Design review of the part built by this model. Coordinates are the model's own, in mm. Face numbers are marked on the shaded views. A direction names the side the tool comes from. Coordinates: 2 decimals unless noted, no trailing zeros. Write each loop counter-clockwise with the first axis right and the second up, starting at its lowest first coordinate (ties: lowest second). Pieces come first, ordered by that corner, then holes. Notation, with made-up numbers: (75.25, 30.25) -> (118.25, 30.25) arc R22 cw to (118.25, 42.25) -> close; hole circle Ø3 at (26.5, 11.25). An arc over 180 degrees is marked (long way). Answer in a Markdown table with one row per item. Add a question column.
Item 1: Clearance check with flat-ended pins moving along their axes: P1, Ø5.5, axis at x = -1.5, y = -1.5, coming from the +Z side; P2, Ø11, axis at x = -1.5, y = -0.5, coming from the +Z side. State where each tip first meets the part, or that it passes through.
Item 2: Take a section at A-A, the plane y = 1.75. Write out the cut boundary in (x, z).
Item 3: For the marked faces 4 and 5, list the 3-axis set-ups (+Z, -Z, +X, -X, +Y, -Y) from which the entire face can be reached by the end or side of a thin tool; tool diameter is ignored.
Item 4: Take a section at C-C, the plane z = 10.55. Write out the cut boundary in (x, y), and give its area (3 significant figures).
Item 5: Take a section at B-B, the plane x = 20. Write out the cut boundary in (y, z).
Item 6: Take a section at D-D, the plane z = 4. Write out the cut boundary in (x, y).
Item 7: To check wall thickness, follow line 1 (X direction, y = 0, z = -15); line 2 (X direction, y = -10.5, z = -3); line 3 (Y direction, x = 0.5, z = -14). State the ranges of each line that lie inside material, in increasing order.
Item 8: Draft analysis for pull direction Y (two halves, no side actions). For the marked faces 1, 2 and 3, state which applies: released by +Y, released by -Y, zero draft, split by the parting line, or undercut.
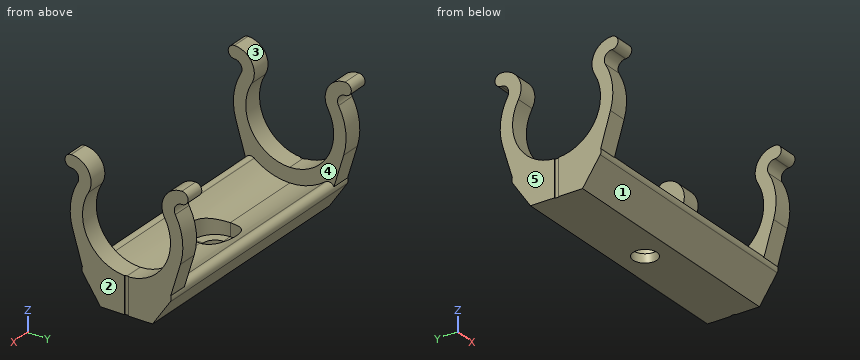
from build123d import *

# Parameters (mm, degrees)
PAD005_DEPTH                  = 29
PAD006_DEPTH                  = 4.5
SKETCH014_R                   = 2.75
POCKET005_DEPTH               = 107.300407
SKETCH015_R                   = 5
POCKET006_DEPTH               = 16.5
PAD005_MIRRORED002_2_DEPTH    = 29
PAD006_MIRRORED002_2_DEPTH    = 4.5
SKETCH014_MIRRORED002_2_R     = 2.75
POCKET005_MIRRORED002_2_DEPTH = 107.300407
SKETCH015_MIRRORED002_2_R     = 5
POCKET006_MIRRORED002_2_DEPTH = 16.5
SKETCH023_W                   = 1
SKETCH023_H                   = 10
POCKET011_DEPTH               = 0.2


with BuildPart() as part:
    # Sketch012 → Pad005 (new body)
    with BuildSketch(Plane.YZ):
        with BuildLine():
            ThreePointArc((0, -13.5), (4.330629, -12.786542), (8.203522, -10.721578))
            ThreePointArc((10.083563, -12.5), (9.900722, -10.810344), (8.203522, -10.721578))
            Line((6, -18.5), (10.083563, -12.5))
            Line((0, -18.5), (6, -18.5))
            Line((0, -13.5), (0, -18.5))
        make_face()
    pad005 = extrude(amount=PAD005_DEPTH)

    # Sketch013 → Pad006 (join)
    with BuildSketch(Plane.YZ.offset(29)):
        with BuildLine():
            ThreePointArc((0, -10.15), (8.790158, -5.075), (8.790158, 5.075))
            ThreePointArc((12.773875, 11.975), (8.790158, 9.675), (8.790158, 5.075))
            ThreePointArc((12.773875, 9.125), (14.198875, 10.55), (12.773875, 11.975))
            ThreePointArc((12.773875, 9.125), (11.25833, 8.25), (11.25833, 6.5))
            ThreePointArc((12.442941, -3.764734), (12.914285, 1.490384), (11.25833, 6.5))
            Line((12.442941, -3.764734), (9.8, -12.5))
            Line((9.8, -12.5), (0, -14.15))
            Line((0, -10.15), (0, -14.15))
        make_face()
    pad006 = extrude(amount=-PAD006_DEPTH)

    # Sketch014 → Pocket005 (cut, through all)
    with BuildSketch(Plane.XY):
        Circle(SKETCH014_R)
    pocket005 = extrude(amount=-POCKET005_DEPTH, mode=Mode.SUBTRACT)

    # Sketch015 → Pocket006 (cut)
    with BuildSketch(Plane.XY):
        Circle(SKETCH015_R)
    pocket006 = extrude(amount=-POCKET006_DEPTH, mode=Mode.SUBTRACT)

    # Sketch012 Mirrored002 2 → Pad005 Mirrored002 2 (add)
    with BuildSketch(Plane(origin=(0, 0, 0), x_dir=(0, -1, 0), z_dir=(-1, 0, 0))):
        with BuildLine():
            ThreePointArc((0, -13.5), (4.330629, -12.786542), (8.203522, -10.721578))
            ThreePointArc((10.083563, -12.5), (9.900722, -10.810344), (8.203522, -10.721578))
            Line((6, -18.5), (10.083563, -12.5))
            Line((0, -18.5), (6, -18.5))
            Line((0, -13.5), (0, -18.5))
        make_face()
    pad005_mirrored002_2 = extrude(amount=-PAD005_MIRRORED002_2_DEPTH)

    # Sketch013 Mirrored002 2 → Pad006 Mirrored002 2 (add)
    with BuildSketch(Plane(origin=(29, 0, 0), x_dir=(0, -1, 0), z_dir=(-1, 0, 0))):
        with BuildLine():
            ThreePointArc((0, -10.15), (8.790158, -5.075), (8.790158, 5.075))
            ThreePointArc((12.773875, 11.975), (8.790158, 9.675), (8.790158, 5.075))
            ThreePointArc((12.773875, 9.125), (14.198875, 10.55), (12.773875, 11.975))
            ThreePointArc((12.773875, 9.125), (11.25833, 8.25), (11.25833, 6.5))
            ThreePointArc((12.442941, -3.764734), (12.914285, 1.490384), (11.25833, 6.5))
            Line((12.442941, -3.764734), (9.8, -12.5))
            Line((9.8, -12.5), (0, -14.15))
            Line((0, -10.15), (0, -14.15))
        make_face()
    pad006_mirrored002_2 = extrude(amount=PAD006_MIRRORED002_2_DEPTH)

    # Sketch014 Mirrored002 2 → Pocket005 Mirrored002 2 (cut, through all)
    with BuildSketch(Plane(origin=(0, 0, 0), x_dir=(1, 0, 0), z_dir=(0, 0, -1))):
        Circle(SKETCH014_MIRRORED002_2_R)
    pocket005_mirrored002_2 = extrude(amount=POCKET005_MIRRORED002_2_DEPTH, mode=Mode.SUBTRACT)

    # Sketch015 Mirrored002 2 → Pocket006 Mirrored002 2 (cut)
    with BuildSketch(Plane(origin=(0, 0, 0), x_dir=(1, 0, 0), z_dir=(0, 0, -1))):
        Circle(SKETCH015_MIRRORED002_2_R)
    pocket006_mirrored002_2 = extrude(amount=POCKET006_MIRRORED002_2_DEPTH, mode=Mode.SUBTRACT)

    # Mirrored003: Pad005, Pad006, Pocket005, Pocket006, Pad005 Mirrored002 2, Pad006 Mirrored002 2, Pocket005 Mirrored002 2, Pocket006 Mirrored002 2 across YZ
    add(pad005.mirror(Plane.YZ))
    add(pad006.mirror(Plane.YZ))
    add(pocket005.mirror(Plane.YZ), mode=Mode.SUBTRACT)
    add(pocket006.mirror(Plane.YZ), mode=Mode.SUBTRACT)
    add(pad005_mirrored002_2.mirror(Plane.YZ))
    add(pad006_mirrored002_2.mirror(Plane.YZ))
    add(pocket005_mirrored002_2.mirror(Plane.YZ), mode=Mode.SUBTRACT)
    add(pocket006_mirrored002_2.mirror(Plane.YZ), mode=Mode.SUBTRACT)

    # Sketch023 → Pocket011 (cut)
    with BuildSketch(Plane.YZ.offset(29)):
        with Locations((0, -15)):
            Rectangle(SKETCH023_W, SKETCH023_H)
    pocket011 = extrude(amount=-POCKET011_DEPTH, mode=Mode.SUBTRACT)

    # Mirrored006: Pocket011 across YZ
    add(pocket011.mirror(Plane.YZ), mode=Mode.SUBTRACT)


solid = part.part
Answers:
| question | item | result |
|---|---|---|
| 1 | P1 | stops at z = -16.5 |
| 1 | P2 | stops at z = -12.09 |
| 2 | outline | (-29, -18.5) -> (-2.12, -18.5) -> (-2.12, -16.5) -> (-4.68, -16.5) -> (-4.68, -13.39) -> (-24.5, -13.39) -> (-24.5, -10) -> (-29, -10) -> close; (2.12, -18.5) -> (29, -18.5) -> (29, -10) -> (24.5, -10) -> (24.5, -13.39) -> (4.68, -13.39) -> (4.68, -16.5) -> (2.12, -16.5) -> close |
| 3 | face 4 | +Z |
| 3 | face 5 | +Z, -Z, -X, +Y, -Y |
| 4 | outline | (-29, -14.2) -> (-24.5, -14.2) -> (-24.5, -9.45) -> (-29, -9.45) -> close; (-29, 9.45) -> (-24.5, 9.45) -> (-24.5, 14.2) -> (-29, 14.2) -> close; (24.5, -14.2) -> (29, -14.2) -> (29, -9.45) -> (24.5, -9.45) -> close; (24.5, 9.45) -> (29, 9.45) -> (29, 14.2) -> (24.5, 14.2) -> close |
| 4 | area | 85.6 mm^2 |
| 5 | outline | (-10.08, -12.5) -> (-6, -18.5) -> (6, -18.5) -> (10.08, -12.5) arc R1.31 ccw to (8.2, -10.72) arc R13.5 cw to (-8.2, -10.72) arc R1.31 ccw to start |
| 6 | outline | (-29, -12.37) -> (-24.5, -12.37) -> (-24.5, -9.33) -> (-29, -9.33) -> close; (-29, 9.33) -> (-24.5, 9.33) -> (-24.5, 12.37) -> (-29, 12.37) -> close; (24.5, -12.37) -> (29, -12.37) -> (29, -9.33) -> (24.5, -9.33) -> close; (24.5, 9.33) -> (29, 9.33) -> (29, 12.37) -> (24.5, 12.37) -> close |
| 7 | line 1 | x = -28.8 to -5, 5 to 28.8 |
| 7 | line 2 | x = -29 to -24.5, 24.5 to 29 |
| 7 | line 3 | y = -9.06 to -4.97, 4.97 to 9.06 |
| 8 | face 1 | released by -Y |
| 8 | face 2 | zero draft |
| 8 | face 3 | undercut |
